Answer from the drawing. Dimensions are ordinates in mm from the lowest x, y and z of the part. A direction names the side the tool comes from. Give positions to 0.01 mm unless a question says otherwise; leave off trailing zeros. Loops run counter-clockwise (first coordinate to the right, second up) from the corner with the lowest first, then second, coordinate; pieces in that order, holes last.
(1) Which of the six approach directions +Z, -Z, +X, -X, +Y, -Y give full straight-line access (tool end or side, diameter ignored) to the marked faces 1 and 2?
(2) This flat-tipped pin is pushed along its axis until it touches: P1, Ø1.2, axis at x = 10.5, y = 34.5, coming from the +Z side. Where does it stop, or does it pass through?
(3) Find section B-B, the plane y = 41. Write down the section's boundary in (x, z), then the cut area to 3 significant figures.
(4) Find section C-C, the plane z = 3. Write down the section's boundary in (x, y), then the cut area to 3 significant figures.
(5) Straight lines are drawn through the part: probe 1 along Y at (x, z) = (4.5, 2.75); probe 2 along Z at (x, y) = (3, 55); probe 3 along X at (y, z) = (22, 1.5). For each, find the intervals that lie inside material, in ascending order.
(6) Determine the mould class of the marked faces 3, 4 and 5 for opening direction Z: pulls with the +Z half, pulls with the -Z half, needs draft (parallel to the pull), parting line crosses it, or undercut.
(7) Find section A-A, the plane x = 5.25. Write down the section's boundary in (y, z), then the cut area to 3 significant figures.
(8) Find section D-D, the plane y = 5.5. Write down the section's boundary in (x, z), then the cut area to 4 significant figures.
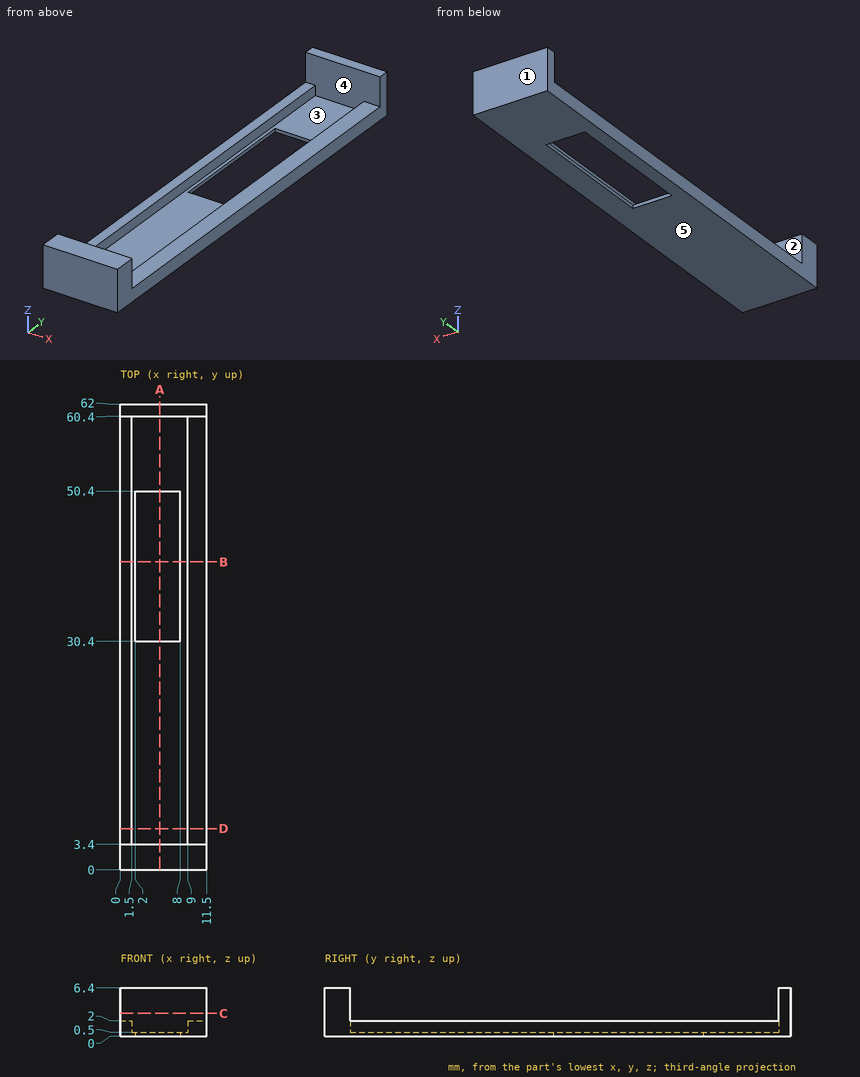
Entries:
1. face 1: +Z, -Z, +X, -X, +Y
1. face 2: +Z
2. P1: stops at z = 2
3. outline: (0, 0) - (2, 0) - (2, 0.5) - (1.5, 0.5) - (1.5, 2) - (0, 2) - close; (8, 0) - (11.5, 0) - (11.5, 2) - (9, 2) - (9, 0.5) - (8, 0.5) - close
3. area: 8.75 mm2
4. outline: (0, 0) - (11.5, 0) - (11.5, 3.4) - (0, 3.4) - close; (0, 60.4) - (11.5, 60.4) - (11.5, 62) - (0, 62) - close
4. area: 57.5 mm2
5. probe 1: y = 0 to 3.4, 60.4 to 62
5. probe 2: z = 0 to 0.5
5. probe 3: x = 0 to 1.5, 9 to 11.5
6. face 3: pulls with the +Z half
6. face 4: needs draft
6. face 5: pulls with the -Z half
7. outline: (0, 0) - (30.4, 0) - (30.4, 0.5) - (3.4, 0.5) - (3.4, 6.4) - (0, 6.4) - close; (50.4, 0) - (62, 0) - (62, 6.4) - (60.4, 6.4) - (60.4, 0.5) - (50.4, 0.5) - close
7. area: 50.5 mm2
8. outline: (0, 0) - (11.5, 0) - (11.5, 2) - (9, 2) - (9, 0.5) - (1.5, 0.5) - (1.5, 2) - (0, 2) - close
8. area: 11.75 mm2
